Verification items for this drawing (mm, ordinates from the low corner). A direction names the side the tool comes from. Round coordinates to 2 decimals unless told otherwise and drop trailing zeros. Loops run counter-clockwise (first coordinate to the right, second up) from the corner with the lowest first, then second, coordinate; pieces in that order, holes last. Notation, with made-up numbers: M 1,-30.5 L 51,-30.5 A14 ccw 51,-18.5 Z; hole C 18.5,-14 d2. An arc over 180 degrees is marked long. One line per item, written item: value.
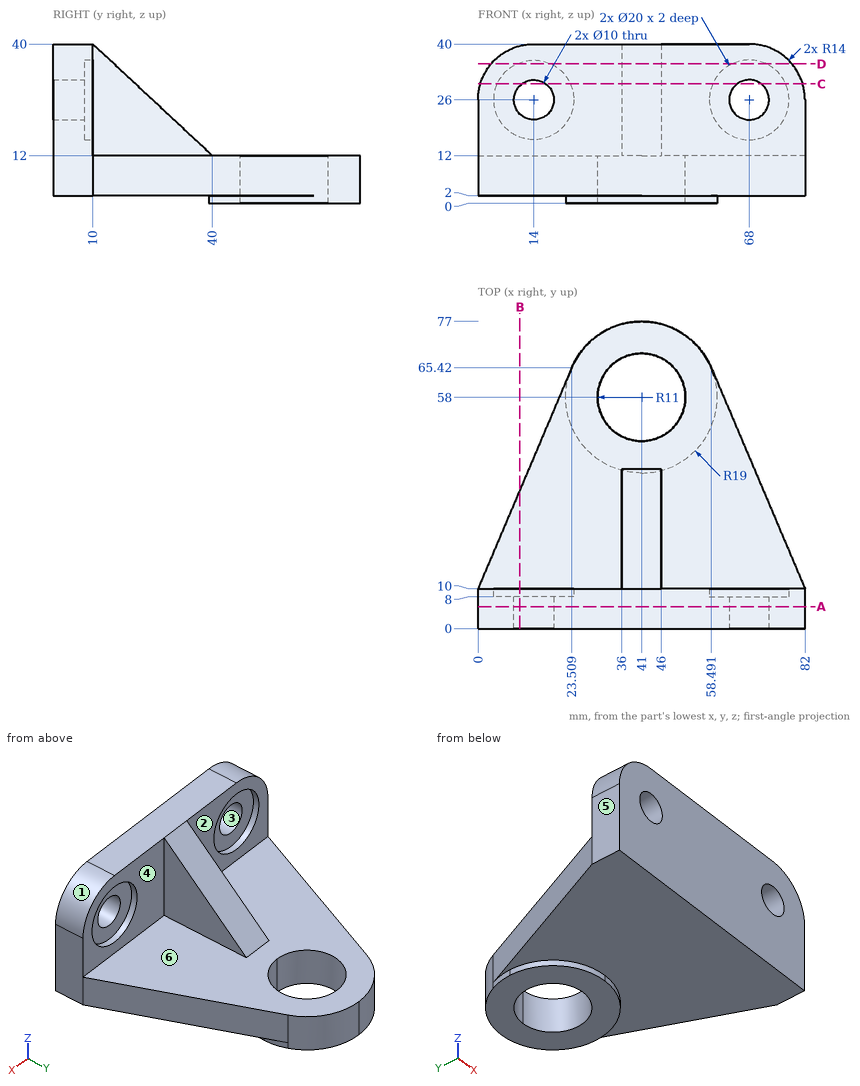
(1) Sectioned sample at D-D on z = 35. Enter the section's corners in (x, y).
Completed:
outline: M 3.28,0 L 78.72,0 L 78.72,10 L 72.36,10 L 72.36,8 L 63.64,8 L 63.64,10 L 46,10 L 46,15.36 L 36,15.36 L 36,10 L 18.36,10 L 18.36,8 L 9.64,8 L 9.64,10 L 3.28,10 Z
(2) Sectioned sample at C-C on z = 30. Enter the section's corners in (x, y) (1 decimal).
Completed:
outline: M 0.6,0 L 11,0 L 11,8 L 4.8,8 L 4.8,10 L 0.6,10 Z; M 17,0 L 65,0 L 65,8 L 58.8,8 L 58.8,10 L 46,10 L 46,20.7 L 36,20.7 L 36,10 L 23.2,10 L 23.2,8 L 17,8 Z; M 71,0 L 81.4,0 L 81.4,10 L 77.2,10 L 77.2,8 L 71,8 Z
(3) Sectioned sample at B-B on x = 10.5. Enter the section's corners in (y, z) (1 decimal).
Completed:
outline: M 0,2 L 34.8,2 L 34.8,12 L 10,12 L 10,16.6 L 8,16.6 L 8,22.4 L 0,22.4 Z; M 0,29.6 L 8,29.6 L 8,35.4 L 10,35.4 L 10,39.6 L 0,39.6 Z
(4) Mould release check, pull along X, two halves, no side actions. Record for the marked faces 1, 2 and 3: +X half, -X half, draft (parallel to the pull), parting line (faces both ways), or undercut.
Completed:
face 1: +X half
face 2: draft
face 3: undercut
(5) Depth check by flat-ended pin: pin 1 Ø8.5 at (y, z) = (28, 29.5) entering from +X; pin 2 Ø4 at (x, z) = (47, 29.5) entering from +Y (1 decimal); pin 3 Ø10 at (x, z) = (10, 28.5) entering from +Y; pin 4 Ø5 at (x, z) = (27.5, 6.5) entering from -Y. Enter the tip coordinate at first touch or a pass-through.
Completed:
pin 1: passes through
pin 2: stops at y = 23.1
pin 3: stops at y = 8
pin 4: stops at y = 0
(6) Sectioned sample at A-A on y = 5.5. Enter the section's corners in (x, z).
Completed:
outline: M 0,2 L 82,2 L 82,26 A14 ccw 68,40 L 14,40 A14 ccw 0,26 Z; hole C 14,26 d10; hole C 68,26 d10
(7) Tool access check on the marked faces 4, 5 and 6. Record the directions out of +Z, -Z, +X, -X, +Y, -Y that give a thin tool (end or side, any length) a straight path to the whole face; none if there is none.
Completed:
face 4: +Z, +X, +Y
face 5: +Z, -Z, -X, +Y, -Y
face 6: +Z, +Y
(8) Thickness scan on L1, parallel to X at y = 8.85, z = 26; L2, parallel to X at y = 5, z = 26; L3, parallel to Z at x = 68, y = 3.5. Record the ranges inside material, lowest first. Write a range as from..to.
Completed:
L1: x = 0..4, 24..58, 78..82
L2: x = 0..9, 19..63, 73..82
L3: z = 2..21, 31..40
